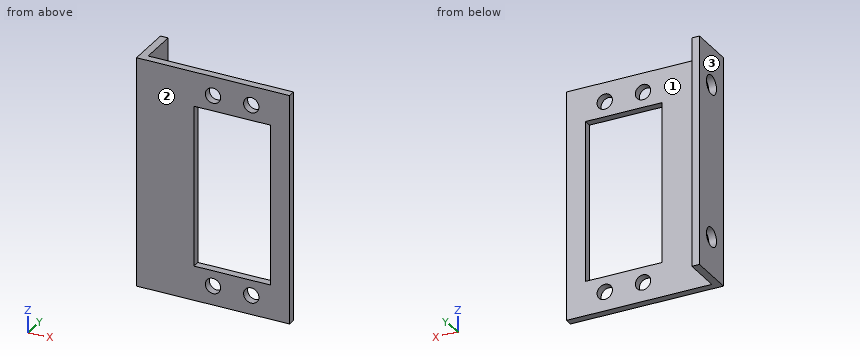
from build123d import *

# Parameters (mm, degrees)
SALIENTE_EXTRUIR1_DEPTH = 60
CROQUIS3_R              = 2.5
CORTAR_EXTRUIR1_DEPTH   = 60
CROQUIS4_R              = 2
CROQUIS4_W              = 20
CROQUIS4_H              = 42
CORTAR_EXTRUIR2_DEPTH   = 60


with BuildPart() as part:
    # Croquis2 → Saliente-Extruir1 (new body)
    with BuildSketch(Plane.XY):
        Polygon((22.222055452, 0), (-17.777944548, 0), (-17.777944548, 12), (-15.777944548, 12), (-15.777944548, 2), (22.222055452, 2), align=None)
    extrude(amount=SALIENTE_EXTRUIR1_DEPTH)

    # Croquis3 → Cortar-Extruir1 (cut)
    with BuildSketch(Plane.ZY.offset(17.777944548)):
        with Locations((10, 6)):
            Circle(CROQUIS3_R)
        with Locations((50, 6)):
            Circle(CROQUIS3_R)
    extrude(amount=-CORTAR_EXTRUIR1_DEPTH, mode=Mode.SUBTRACT)

    # Croquis4 → Cortar-Extruir2 (cut)
    with BuildSketch(Plane.XZ):
        with Locations((2.222055452, 55)):
            Circle(CROQUIS4_R)
        with Locations((12.222055452, 55)):
            Circle(CROQUIS4_R)
        with Locations((2.222055452, 5)):
            Circle(CROQUIS4_R)
        with Locations((12.222055452, 5)):
            Circle(CROQUIS4_R)
        with Locations((7.222055452, 30)):
            Rectangle(CROQUIS4_W, CROQUIS4_H)
    extrude(amount=-CORTAR_EXTRUIR2_DEPTH, mode=Mode.SUBTRACT)


solid = part.part
Build history of the part. All positions in model axes, mm. Face numbers are marked on the shaded views. Give positions to 0.01 mm unless a question says otherwise; leave off trailing zeros. Order: outer loops, then holes, each group sorted by start corner. A loop starts at its lowest first (then second) coordinate and runs counter-clockwise, first axis right, second up. Notation, with made-up numbers: M 59.5,11 L 99.5,11 A28 ccw 99.5,47 Z; hole C -1.75,11 d6. An arc over 180 degrees is marked long. Put each result on its own line as item: value.
Item 1: Cut at C-C on z = 20. Write the cut outline in (x, y).
Results are:
outline: M -17.78,0 L -2.78,0 L -2.78,2 L -15.78,2 L -15.78,12 L -17.78,12 Z; M 17.22,0 L 22.22,0 L 22.22,2 L 17.22,2 Z
Item 2: Drop flat-ended pins along their axis: pin 1 Ø3 at (y, z) = (7, 18.5) entering from +X; pin 2 Ø5 at (x, z) = (-4, 19) entering from +Y. Give the stop position or say it passes through.
Results are:
pin 1: x = -15.78
pin 2: y = 2
Item 3: Cut at D-D on y = 6. Write the cut outline in (x, z).
Results are:
outline: M -17.78,0 L -15.78,0 L -15.78,7.5 L -17.78,7.5 Z; M -17.78,12.5 L -15.78,12.5 L -15.78,47.5 L -17.78,47.5 Z; M -17.78,52.5 L -15.78,52.5 L -15.78,60 L -17.78,60 Z
Item 4: Wall check: probe 1 along Z at (x, y) = (17, 1.5); probe 2 along X at (y, z) = (1.5, 16); probe 3 along Y at (x, z) = (-16, 50). Give the ranges that are in metal, low to high.
Results are:
probe 1: 0 to 9, 51 to 60
probe 2: -17.78 to -2.78, 17.22 to 22.22
probe 3: 0 to 3.5, 8.5 to 12
Item 5: Cut at A-A on z = 5. Write the cut outline in (x, y).
Results are:
outline: M -17.78,0 L 0.22,0 L 0.22,2 L -15.78,2 L -15.78,12 L -17.78,12 Z; M 4.22,0 L 10.22,0 L 10.22,2 L 4.22,2 Z; M 14.22,0 L 22.22,0 L 22.22,2 L 14.22,2 Z
Item 6: Pull direction Y, two halves, no side cores. Call the marked faces 1, 2 and 3: +Y half, -Y half, draft (parallel to the pull), parting line (faces both ways), or undercut.
Results are:
face 1: +Y half
face 2: -Y half
face 3: draft
Item 7: Cut at B-B on x = -0.5. Write the cut outline in (y, z).
Results are:
outline: M 0,0 L 2,0 L 2,9 L 0,9 Z; M 0,51 L 2,51 L 2,60 L 0,60 Z
